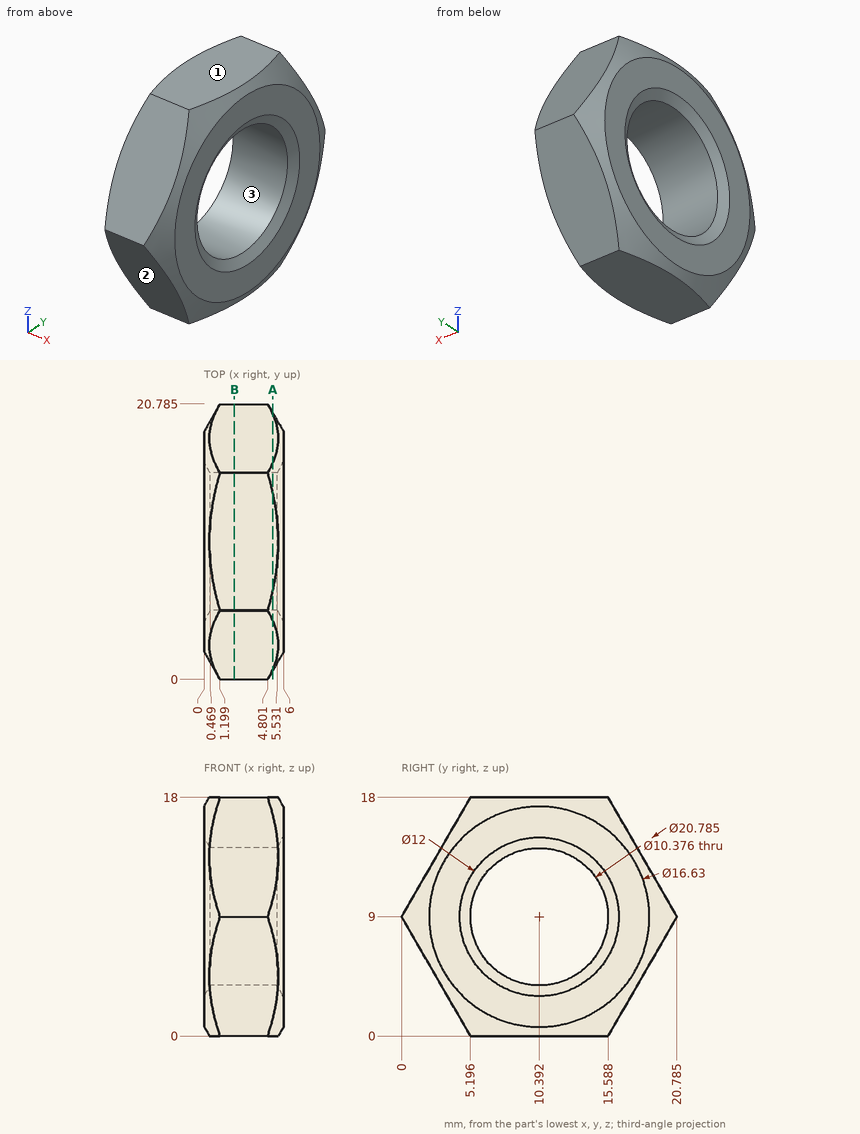
Verification items for this drawing (mm, ordinates from the low corner). Give positions to 0.01 mm unless a question says otherwise; leave off trailing zeros. Write each loop counter-clockwise with the first axis right and the second up, starting at its lowest first coordinate (ties: lowest second). Pieces come first, ordered by that corner, then holes.
1) Cross-section at A-A (x = 5.2). Record the boundary of the cut face in (y, z) (1 decimal).
Values follow:
outline: (0.8, 7.6) - (4.4, 1.4) arc R9.7 ccw to (6.8, 0) - (14, 0) arc R9.7 ccw to (16.4, 1.4) - (20, 7.6) arc R9.7 ccw to (20, 10.4) - (16.4, 16.6) arc R9.7 ccw to (14, 18) - (6.8, 18) arc R9.7 ccw to (4.4, 16.6) - (0.8, 10.4) arc R9.7 ccw to start; hole circle Ø10.4 at (10.4, 9)
2) Release check for a two-part mould opening along Z. For the marked faces 1, 2 and 3 record: released by +Z, released by -Z, zero draft, split by the parting line, or undercut.
Values follow:
face 1: released by +Z
face 2: released by -Z
face 3: undercut
3) Cross-section at B-B (x = 2.3). Record the boundary of the cut face in (y, z) (1 decimal), plus the area to 3 significant figures.
Values follow:
outline: (0, 9) - (5.2, 0) - (15.6, 0) - (20.8, 9) - (15.6, 18) - (5.2, 18) - close; hole circle Ø10.4 at (10.4, 9)
area: 196 mm2
4) Go/stop test with flat-tipped pins: pin 1 Ø2 at (y, z) = (11, 5) entering from +X; pin 2 Ø1.5 at (x, z) = (4.5, 15.5) entering from +Y (1 decimal). Record where each tip stops, or that it passes through.
Values follow:
pin 1: passes through
pin 2: stops at y = 17.5
5) Thickness scan on line 1 (Z direction, x = 4.8, y = 15) (1 decimal); line 2 (Y direction, x = 2.45, z = 4.5) (1 decimal); line 3 (Y direction, x = 5.1, z = 8.75) (1 decimal). Record the ranges inside material, lowest first.
Values follow:
line 1: z = 0 to 6.6, 11.4 to 18
line 2: y = 2.6 to 7.8, 13 to 18.2
line 3: y = 0.5 to 5.2, 15.6 to 20.3
